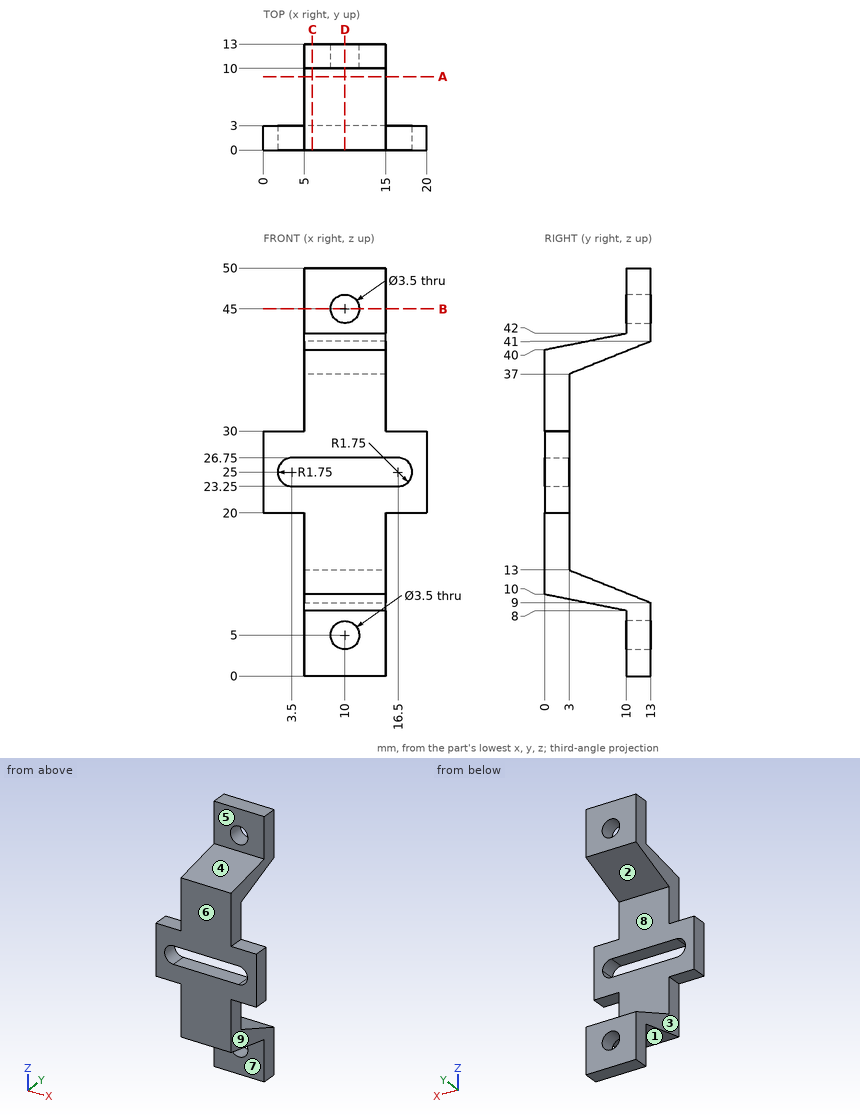
Verification items for this drawing (mm, ordinates from the low corner). A direction names the side the tool comes from. Give positions to 0.01 mm unless a question says otherwise; leave off trailing zeros. Write each loop counter-clockwise with the first axis right and the second up, starting at its lowest first coordinate (ties: lowest second). Pieces come first, ordered by that corner, then holes.
1) Cross-section at B-B (z = 45). Record the boundary of the cut face in (x, y), plus the area to 3 significant figures.
Values follow:
outline: (5, 10) - (8.25, 10) - (8.25, 13) - (5, 13) - close; (11.75, 10) - (15, 10) - (15, 13) - (11.75, 13) - close
area: 19.5 mm2
2) Set-up check for the marked faces 5, 6, 7, 8 and 9: record each of +Z, -Z, +X, -X, +Y, -Y from which the full face is reachable in a straight line by a thin tool's end or side.
Values follow:
face 5: +Z, +X, -X, -Y
face 6: +Z, -Z, +X, -X, -Y
face 7: -Z, +X, -X, -Y
face 8: +X, -X, +Y
face 9: -Z, +X, +Y, -Y
3) Thickness scan on line 1 (X direction, y = 11.45, z = 45); line 2 (Z direction, x = 14.5, y = 10.5); line 3 (Y direction, x = 6.25, z = 4.5). Record the ranges inside material, lowest first.
Values follow:
line 1: x = 5 to 8.25, 11.75 to 15
line 2: z = 0 to 10, 40 to 50
line 3: y = 10 to 13
4) Go/stop test with flat-tipped pins: pin 1 Ø2.5 at (x, y) = (9, 1) entering from +Z; pin 2 Ø1.5 at (x, y) = (1.5, 1.5) entering from -Z; pin 3 Ø6.5 at (y, z) = (7, 7.5) entering from +X. Record where each tip stops, or that it passes through.
Values follow:
pin 1: stops at z = 40.45
pin 2: stops at z = 20
pin 3: stops at x = 15
5) Cross-section at D-D (x = 10). Record the boundary of the cut face in (y, z), plus the area to 4 significant figures.
Values follow:
outline: (0, 10) - (10, 8) - (10, 6.75) - (13, 6.75) - (13, 9) - (3, 13) - (3, 23.25) - (0, 23.25) - close; (0, 26.75) - (3, 26.75) - (3, 37) - (13, 41) - (13, 43.25) - (10, 43.25) - (10, 42) - (0, 40) - close; (10, 0) - (13, 0) - (13, 3.25) - (10, 3.25) - close; (10, 46.75) - (13, 46.75) - (13, 50) - (10, 50) - close
area: 158.5 mm2
6) Cross-section at A-A (y = 9). Record the boundary of the cut face in (x, z).
Values follow:
outline: (5, 8.2) - (15, 8.2) - (15, 10.6) - (5, 10.6) - close; (5, 39.4) - (15, 39.4) - (15, 41.8) - (5, 41.8) - close
7) Release check for a two-part mould opening along Z. For the marked faces 1, 2, 3 and 4 record: released by +Z, released by -Z, zero draft, split by the parting line, or undercut.
Values follow:
face 1: released by -Z
face 2: undercut
face 3: zero draft
face 4: released by +Z
8) Cross-section at C-C (x = 6). Record the boundary of the cut face in (y, z), plus the area to 4 significant figures.
Values follow:
outline: (0, 10) - (10, 8) - (10, 0) - (13, 0) - (13, 9) - (3, 13) - (3, 23.25) - (0, 23.25) - close; (0, 26.75) - (3, 26.75) - (3, 37) - (13, 41) - (13, 50) - (10, 50) - (10, 42) - (0, 40) - close
area: 179.5 mm2
